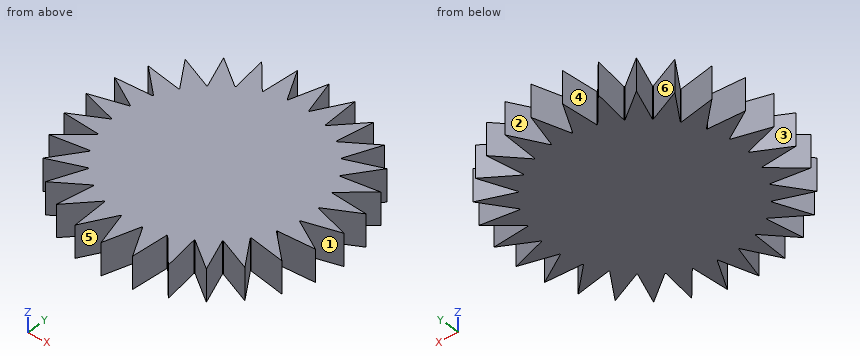
Autodesk Inventor part; units mm, degrees
ref_plane "YZ Plane" through (0, 0, 0) normal (1, 0, 0) x (0, 1, 0)
ref_plane "XZ Plane" through (0, 0, 0) normal (0, 1, 0) x (-1, 0, 0)
ref_plane "XY Plane" through (0, 0, 0) normal (0, 0, 1) x (1, 0, 0)
sketch "Sketch3" plane through (0, 0, 0) normal (0, 0, 1) x (1, 0, 0)
  line L0 (-5.1387, 1.3261) -> (-4.3137, 4.1201)
  line L1 (-4.3137, 4.1201) -> (-3.4886, 1.3261)
  line L2 (-4.3137, 1.3261) -> (-5.1387, 1.3261) construction
  line L3 (-4.3137, 1.3261) -> (-4.3137, 1.6791) construction
  circle A0 centre (-4.3137, -6.2491) radius 7.62 construction
  circle A1 centre (-4.3137, -6.2491) radius 7.62 construction
  line L4 (-6.8037, 0.9526) -> (-6.621, 3.8601)
  line L5 (-6.621, 3.8601) -> (-5.1949, 1.3198)
  circle A2 centre (-4.3137, -6.2491) radius 7.62 construction
  line L6 (-8.3438, 0.218) -> (-8.8127, 3.0933)
  line L7 (-8.8127, 3.0933) -> (-6.8571, 0.9339)
  circle A3 centre (-4.3137, -6.2491) radius 7.62 construction
  line L8 (-9.6818, -0.841) -> (-10.7788, 1.8579)
  line L9 (-10.7788, 1.8579) -> (-8.3917, 0.1879)
  circle A4 centre (-4.3137, -6.2491) radius 7.62 construction
  line L10 (-10.7506, -2.1711) -> (-12.4206, 0.216)
  line L11 (-12.4206, 0.216) -> (-9.7218, -0.881)
  circle A5 centre (-4.3137, -6.2491) radius 7.62 construction
  line L12 (-11.4967, -3.7057) -> (-13.656, -1.75)
  line L13 (-13.656, -1.75) -> (-10.7807, -2.219)
  circle A6 centre (-4.3137, -6.2491) radius 7.62 construction
  line L14 (-11.8825, -5.3678) -> (-14.4229, -3.9417)
  line L15 (-14.4229, -3.9417) -> (-11.5154, -3.7591)
  circle A7 centre (-4.3137, -6.2491) radius 7.62 construction
  line L16 (-11.8889, -7.0741) -> (-14.6829, -6.2491)
  line L17 (-14.6829, -6.2491) -> (-11.8889, -5.424)
  circle A8 centre (-4.3137, -6.2491) radius 7.62 construction
  line L18 (-11.5154, -8.7391) -> (-14.4229, -8.5564)
  line L19 (-14.4229, -8.5564) -> (-11.8825, -7.1303)
  circle A9 centre (-4.3137, -6.2491) radius 7.62 construction
  line L20 (-10.7807, -10.2792) -> (-13.656, -10.7481)
  line L21 (-13.656, -10.7481) -> (-11.4967, -8.7925)
  circle A10 centre (-4.3137, -6.2491) radius 7.62 construction
  line L22 (-9.7218, -11.6172) -> (-12.4206, -12.7142)
  line L23 (-12.4206, -12.7142) -> (-10.7506, -10.3271)
  circle A11 centre (-4.3137, -6.2491) radius 7.62 construction
  line L24 (-8.3917, -12.686) -> (-10.7788, -14.356)
  line L25 (-10.7788, -14.356) -> (-9.6818, -11.6572)
  circle A12 centre (-4.3137, -6.2491) radius 7.62 construction
  line L26 (-6.8571, -13.4321) -> (-8.8127, -15.5914)
  line L27 (-8.8127, -15.5914) -> (-8.3438, -12.7161)
  circle A13 centre (-4.3137, -6.2491) radius 7.62 construction
  line L28 (-5.1949, -13.8179) -> (-6.621, -16.3583)
  line L29 (-6.621, -16.3583) -> (-6.8037, -13.4508)
  circle A14 centre (-4.3137, -6.2491) radius 7.62 construction
  line L30 (-3.4886, -13.8243) -> (-4.3137, -16.6183)
  line L31 (-4.3137, -16.6183) -> (-5.1387, -13.8243)
  circle A15 centre (-4.3137, -6.2491) radius 7.62 construction
  line L32 (-1.8237, -13.4508) -> (-2.0063, -16.3583)
  line L33 (-2.0063, -16.3583) -> (-3.4324, -13.8179)
  circle A16 centre (-4.3137, -6.2491) radius 7.62 construction
  line L34 (-0.2836, -12.7161) -> (0.1853, -15.5914)
  line L35 (0.1853, -15.5914) -> (-1.7703, -13.4321)
  circle A17 centre (-4.3137, -6.2491) radius 7.62 construction
  line L36 (1.0544, -11.6572) -> (2.1514, -14.356)
  line L37 (2.1514, -14.356) -> (-0.2357, -12.686)
  circle A18 centre (-4.3137, -6.2491) radius 7.62 construction
  line L38 (2.1233, -10.3271) -> (3.7933, -12.7142)
  line L39 (3.7933, -12.7142) -> (1.0944, -11.6172)
  circle A19 centre (-4.3137, -6.2491) radius 7.62 construction
  line L40 (2.8693, -8.7925) -> (5.0286, -10.7481)
  line L41 (5.0286, -10.7481) -> (2.1534, -10.2792)
  circle A20 centre (-4.3137, -6.2491) radius 7.62 construction
  line L42 (3.2552, -7.1303) -> (5.7955, -8.5564)
  line L43 (5.7955, -8.5564) -> (2.888, -8.7391)
  circle A21 centre (-4.3137, -6.2491) radius 7.62 construction
  line L44 (3.2615, -5.424) -> (6.0555, -6.2491)
  line L45 (6.0555, -6.2491) -> (3.2615, -7.0741)
  circle A22 centre (-4.3137, -6.2491) radius 7.62 construction
  line L46 (2.888, -3.7591) -> (5.7955, -3.9417)
  line L47 (5.7955, -3.9417) -> (3.2552, -5.3678)
  circle A23 centre (-4.3137, -6.2491) radius 7.62 construction
  line L48 (2.1534, -2.219) -> (5.0286, -1.75)
  line L49 (5.0286, -1.75) -> (2.8693, -3.7057)
  circle A24 centre (-4.3137, -6.2491) radius 7.62 construction
  line L50 (1.0944, -0.881) -> (3.7933, 0.216)
  line L51 (3.7933, 0.216) -> (2.1233, -2.1711)
  circle A25 centre (-4.3137, -6.2491) radius 7.62 construction
  line L52 (-0.2357, 0.1879) -> (2.1514, 1.8579)
  line L53 (2.1514, 1.8579) -> (1.0544, -0.841)
  circle A26 centre (-4.3137, -6.2491) radius 7.62 construction
  line L54 (-1.7703, 0.9339) -> (0.1853, 3.0933)
  line L55 (0.1853, 3.0933) -> (-0.2836, 0.218)
  circle A27 centre (-4.3137, -6.2491) radius 7.62 construction
  line L56 (-3.4324, 1.3198) -> (-2.0063, 3.8601)
  line L57 (-2.0063, 3.8601) -> (-1.8237, 0.9526)
  arc A28 (-10.7506, -2.1711) -> (-10.7807, -2.219) centre (-4.3137, -6.2491) ccw
  arc A29 (-11.4967, -3.7057) -> (-11.5154, -3.7591) centre (-4.3137, -6.2491) ccw
  arc A30 (-11.8825, -5.3678) -> (-11.8889, -5.424) centre (-4.3137, -6.2491) ccw
  arc A31 (-11.8889, -7.0741) -> (-11.8825, -7.1303) centre (-4.3137, -6.2491) ccw
  arc A32 (-11.5154, -8.7391) -> (-11.4967, -8.7925) centre (-4.3137, -6.2491) ccw
  arc A33 (-10.7807, -10.2792) -> (-10.7506, -10.3271) centre (-4.3137, -6.2491) ccw
  arc A34 (-9.7218, -11.6172) -> (-9.6818, -11.6572) centre (-4.3137, -6.2491) ccw
  arc A35 (-8.3917, -12.686) -> (-8.3438, -12.7161) centre (-4.3137, -6.2491) ccw
  arc A36 (-6.8571, -13.4321) -> (-6.8037, -13.4508) centre (-4.3137, -6.2491) ccw
  arc A37 (-5.1949, -13.8179) -> (-5.1387, -13.8243) centre (-4.3137, -6.2491) ccw
  arc A38 (-3.4886, -13.8243) -> (-3.4324, -13.8179) centre (-4.3137, -6.2491) ccw
  arc A39 (-1.8237, -13.4508) -> (-1.7703, -13.4321) centre (-4.3137, -6.2491) ccw
  arc A40 (-0.2836, -12.7161) -> (-0.2357, -12.686) centre (-4.3137, -6.2491) ccw
  arc A41 (1.0544, -11.6572) -> (1.0944, -11.6172) centre (-4.3137, -6.2491) ccw
  arc A42 (2.1233, -10.3271) -> (2.1534, -10.2792) centre (-4.3137, -6.2491) ccw
  arc A43 (2.8693, -8.7925) -> (2.888, -8.7391) centre (-4.3137, -6.2491) ccw
  arc A44 (3.2552, -7.1303) -> (3.2615, -7.0741) centre (-4.3137, -6.2491) ccw
  arc A45 (3.2615, -5.424) -> (3.2552, -5.3678) centre (-4.3137, -6.2491) ccw
  arc A46 (2.888, -3.7591) -> (2.8693, -3.7057) centre (-4.3137, -6.2491) ccw
  arc A47 (2.1534, -2.219) -> (2.1233, -2.1711) centre (-4.3137, -6.2491) ccw
  arc A48 (1.0944, -0.881) -> (1.0544, -0.841) centre (-4.3137, -6.2491) ccw
  arc A49 (-0.2357, 0.1879) -> (-0.2836, 0.218) centre (-4.3137, -6.2491) ccw
  arc A50 (-1.7703, 0.9339) -> (-1.8237, 0.9526) centre (-4.3137, -6.2491) ccw
  arc A51 (-3.4324, 1.3198) -> (-3.4886, 1.3261) centre (-4.3137, -6.2491) ccw
  arc A52 (-5.1387, 1.3261) -> (-5.1949, 1.3198) centre (-4.3137, -6.2491) ccw
  arc A53 (-6.8037, 0.9526) -> (-6.8571, 0.9339) centre (-4.3137, -6.2491) ccw
  arc A54 (-8.3438, 0.218) -> (-8.3917, 0.1879) centre (-4.3137, -6.2491) ccw
  arc A55 (-9.6818, -0.841) -> (-9.7218, -0.881) centre (-4.3137, -6.2491) ccw
  point P0 (0, 0)
  dimension "d21" = 1.6501
  dimension "d22" = 2.794
  dimension "d23" = 15.24
  dimension "d26" = 360
extrude "Extrusion3" add sketch "Sketch3" along normal blind 2.54
properties part number "Big Gear Phone Case Mech"
Here's how the part is built. I have some questions about the finished solid (model axes, mm). Face numbers are marked on the shaded views. A direction names the side the tool comes from. Give positions to 0.01 mm unless a question says otherwise; leave off trailing zeros. Loops run counter-clockwise (first coordinate to the right, second up) from the corner with the lowest first, then second, coordinate; pieces in that order, holes last. Notation, with made-up numbers: (55, 14.5) -> (110, 14.5) arc R29 ccw to (110, 36.5) -> close; hole circle Ø6 at (34, 41). An arc over 180 degrees is marked (long way). Answer as a JSON object with one key per item and string values. Group by question number.
Item 1: Thinking about a two-plate mould opening in X: for the marked faces 1, 2 and 3, which applies, pulls with the +X half, pulls with the -X half, needs draft (parallel to the pull), parting line crosses it, or undercut?
Item 2: Will this pin go through, and if not, where does the flat tip stop? pin 1 (5 mm diameter, centred on x = -9.5, y = -13, fed in from -Z).
Item 3: On a 3-axis mill with a long thin cutter (end or side, diameter ignored), from which of +Z, -Z, +X, -X, +Y, -Y can I reach the whole of each face in a straight line? I mean the marked faces 4, 5 and 6. Say none if no direction works.
Item 4: Imagine slicing it at C-C on y = -5.75. Write out the boundary of the cut face in (x, z), then the cut area to 3 significant figures.
Item 5: Imagine slicing it at A-A on x = 3.5. Write out the boundary of the cut face in (y, z), then the cut area to 3 significant figures.
Item 6: Imagine slicing it at B-B on x = -12.75. Write out the boundary of the cut face in (y, z), then the cut area to 3 significant figures.
Item 7: Imagine slicing it at D-D on x = -6.25. Write out the boundary of the cut face in (y, z), then the cut area to 3 significant figures.
Item 8: I need wall thicknesses on L1, parallel to X at y = -12, z = 2.4; L2, parallel to X at y = -15, z = 0.65; L3, parallel to X at y = -0.25, z = 2.35. Which ranges of each line are inside material? Lowest first, please.
Answer list:
{
 "1": {"face 1": "pulls with the +X half", "face 2": "undercut", "face 3": "pulls with the -X half"},
 "2": {"pin 1": "stops at z = 0"},
 "3": {"face 4": "+Z, -Z, +Y", "face 5": "+Z, -Z, -Y", "face 6": "+Z, -Z"},
 "4": {"outline": "(-12.99, 0) -> (4.37, 0) -> (4.37, 2.54) -> (-12.99, 2.54) -> close", "area": "44.1 mm2"},
 "5": {"outline": "(-12.59, 0) -> (-12.29, 0) -> (-12.29, 2.54) -> (-12.59, 2.54) -> close; (-10.5, 0) -> (-9.36, 0) -> (-9.36, 2.54) -> (-10.5, 2.54) -> close; (-8.7, 0) -> (-7.27, 0) -> (-7.27, 2.54) -> (-8.7, 2.54) -> close; (-7, 0) -> (-5.49, 0) -> (-5.49, 2.54) -> (-7, 2.54) -> close; (-5.23, 0) -> (-3.8, 0) -> (-3.8, 2.54) -> (-5.23, 2.54) -> close; (-3.13, 0) -> (-2, 0) -> (-2, 2.54) -> (-3.13, 2.54) -> close; (-0.2, 0) -> (0.1, 0) -> (0.1, 2.54) -> (-0.2, 2.54) -> close", "area": "18.4 mm2"},
 "6": {"outline": "(-10.6, 0) -> (-9.93, 0) -> (-9.93, 2.54) -> (-10.6, 2.54) -> close; (-8.66, 0) -> (-7.62, 0) -> (-7.62, 2.54) -> (-8.66, 2.54) -> close; (-6.82, 0) -> (-5.68, 0) -> (-5.68, 2.54) -> (-6.82, 2.54) -> close; (-4.88, 0) -> (-3.84, 0) -> (-3.84, 2.54) -> (-4.88, 2.54) -> close; (-2.57, 0) -> (-1.9, 0) -> (-1.9, 2.54) -> (-2.57, 2.54) -> close", "area": "11.6 mm2"},
 "7": {"outline": "(-15.7, 0) -> (3.2, 0) -> (3.2, 2.54) -> (-15.7, 2.54) -> close", "area": "48.0 mm2"},
 "8": {"L1": "x = -11.92 to -10.66, -9.82 to 1.19, 2.04 to 3.29", "L2": "x = -8.72 to -8.28, -6.71 to -5.86, -4.79 to -3.84, -2.77 to -1.92, -0.35 to 0.09", "L3": "x = -12.09 to -11.27, -9.92 to 1.29, 2.65 to 3.47"}
}
